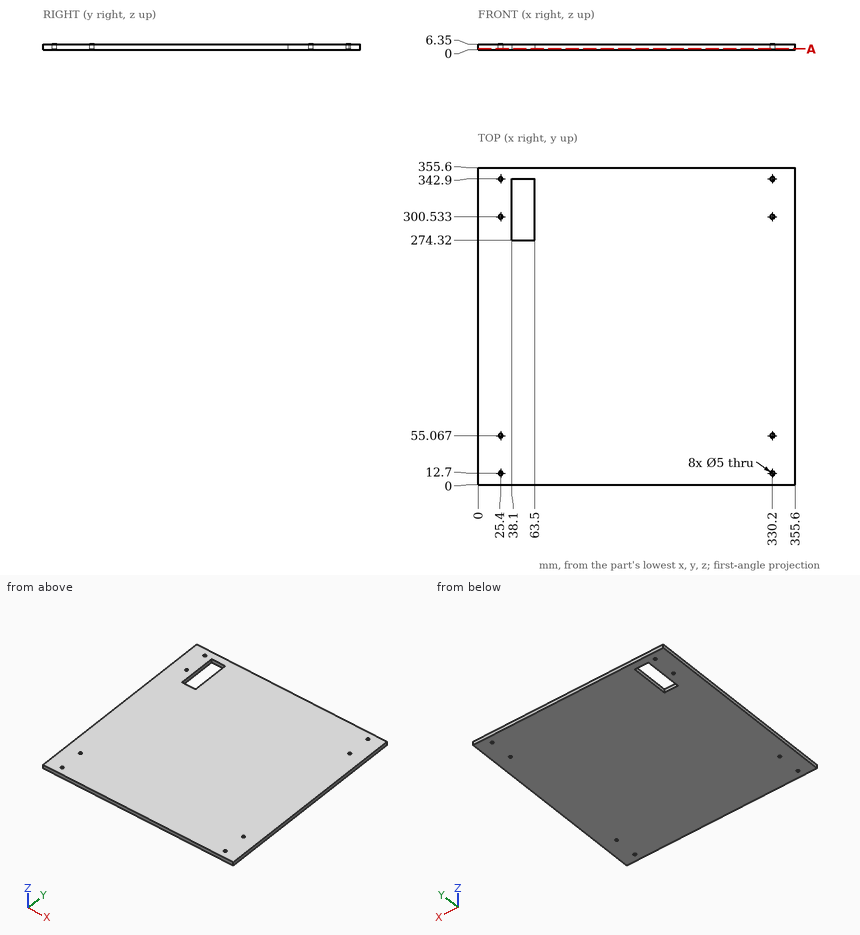
Part print with two shaded views. Sizes in mm from the minimum x, y, z corner. Round coordinates to 2 decimals unless told otherwise and drop trailing zeros. Put each result on its own line as item: value. Start each with the question number.
1) Drill centre lines: probe 1 along Y at (x, z) = (330.2, 4.5); probe 2 along X at (y, z) = (285, 6). Where is each one in solid material? Low to high. Write a range as [from, to].
2) Saw through at A-A, the plane z = 1. Count the separate pieces of the cut face and the enclosed holes in it, and give its area (3 significant figures).
3) Pin check, flat tip, straight feed: pin 1 Ø4 at (x, y) = (25.4, 12.7) entering from +Z. Stop position of the tip, or through.
Resolved:
1. probe 1: [0, 10.2], [15.2, 52.57], [57.57, 298.03], [303.03, 340.4], [345.4, 355.6]
1. probe 2: [0, 38.1], [63.5, 355.6]
2. separate pieces: 1
2. enclosed holes: 9
2. area: 125,000 mm²
3. pin 1: through
